Input: part model. Units: mm. Frame: model coordinates. A direction names the side the tool comes from. Give positions to 0.01 mm unless a question says otherwise; leave off trailing zeros. Loops run counter-clockwise (first coordinate to the right, second up) from the corner with the lowest first, then second, coordinate; pieces in that order, holes last. Notation, with made-up numbers: M -38,19.25 L 12,19.25 A35 cw 12,57.25 Z; hole C -34,60 d1. An arc over 180 degrees is marked long. Answer as a JSON object with one key per item and string values. Group by question number.
1) Section query A-A on y = -1.3. Count the separate pieces of the cut face and the enclosed holes in it, plus the area to 3 significant figures.
2) Ray query, L1, parallel to X at y = 0.15, z = 5; L2, parallel to Z at x = 5.1, y = 1.15; L3, parallel to X at y = 0.45, z = 0.75. Return the intervals inside material, ascending.
3) First-contact query: P1, Ø1, axis at y = 1, z = 4, coming from the -X side; P2, Ø2, axis at y = -1, z = 5, coming from the +X side; P3, Ø3, axis at x = 5.1, z = 3.5, coming from the -Y side. Flat tips, straight axial feed; report the tip coordinate or a pass-through.
4) Access query for faces 5 (the flat face through (-2.35, -1, 3)), 6 (the flat face through (3, -2.5, 3)). Directions: +Z, -Z, +X, -X, +Y, -Y. A direction counts if a zero-diameter tool reaches every point of the face in a straight line with its end or side. Return the directions, or none.
5) Draft query along X for faces 1 (the flat face through (2.35, -1, 3)), 2 (the flat face through (-4.35, -1, 3)), 3 (the flat face through (0.9, 2.4, 7)), 4 (the cylindrical face through (6.8, 0.5, 1)). Return one class per face: +X half, -X half, draft (parallel to the pull), parting line (faces both ways), or undercut.
6) Section query B-B on z = 2. Return loops of the section in (x, y), plus the area to 3 significant figures.
7) Section query C-C on x = 5.1. Return loops of the section in (y, z), plus the area to 3 significant figures.
from build123d import *

# Parameters (mm, degrees)
F1_DEPTH = 7
F2_R     = 1.75
F3_DEPTH = 5.85
F4_R     = 3.49999
F5_R     = 3


# Not quite as in the source:
# - a fillet or chamfer is up to 0.001 mm smaller than in the source, because OpenCascade refuses the exact size


with BuildPart() as f1:
    # F0 (on Top) → F1 (new body)
    with BuildSketch(Plane.XY):
        with BuildLine():
            ThreePointArc((-2.35, 0), (0, 2.35), (2.35, 0))
            Line((2.35, 0), (2.35, -2.5))
            Line((2.35, -2.5), (7.85, -2.5))
            Line((7.85, -2.5), (7.85, 3.35))
            Line((7.85, 3.35), (-4.35, 3.35))
            Line((-4.35, 3.35), (-4.35, -2.5))
            Line((-4.35, -2.5), (-2.35, -2.5))
            Line((-2.35, -2.5), (-2.35, 0))
        make_face()
    extrude(amount=F1_DEPTH)

    # F2 (on face) → F3 (cut, through all)
    with BuildSketch(Plane(origin=(0, 3.35, 0), x_dir=(-1, 0, 0), z_dir=(0, 1, 0))):
        with Locations((-5.1, 3.5)):
            Circle(F2_R)
    extrude(amount=-F3_DEPTH, mode=Mode.SUBTRACT)

    # F4 (radius 3.5 in the source; OpenCascade refuses exactly that, so slightly less here)
    f4_edges = [f1.edges().sort_by_distance(p)[0] for p in [
        (7.85, 0.425, 7),
        (7.85, 0.425, 0),
    ]]
    fillet(f4_edges, radius=F4_R)

    # F5
    f5_edges = [f1.edges().sort_by_distance(p)[0] for p in [
        (-4.35, 3.35, 3.5),
    ]]
    fillet(f5_edges, radius=F5_R)


solid = f1.part
Output:
{
 "1": {"separate pieces": "2", "enclosed holes": "1", "area": "37.6 mm^2"},
 "2": {"L1": "x = -4.35 to -2.35, 2.35 to 4.2, 6 to 7.51", "L2": "z = 0.08 to 1.75, 5.25 to 6.92", "L3": "x = -4.35 to -2.31, 2.31 to 6.52"},
 "3": {"P1": "stops at x = -4.35", "P2": "stops at x = 7.81", "P3": "passes through"},
 "4": {"face 5": "+Z, -Z, -Y", "face 6": "+Z, -Z, +X, -X, -Y"},
 "5": {"face 1": "undercut", "face 2": "-X half", "face 3": "draft", "face 4": "+X half"},
 "6": {"outline": "M -4.35,-2.5 L -2.35,-2.5 L -2.35,0 A2.35 cw 2.35,0 L 2.35,-2.5 L 4.2,-2.5 L 4.2,3.35 L -1.35,3.35 A3 ccw -4.35,0.35 Z; M 6,-2.5 L 7.51,-2.5 L 7.51,3.35 L 6,3.35 Z", "area": "36.5 mm^2"},
 "7": {"outline": "M -2.5,0.08 L 3.35,0.08 L 3.35,1.75 L -2.5,1.75 Z; M -2.5,5.25 L 3.35,5.25 L 3.35,6.92 L -2.5,6.92 Z", "area": "19.5 mm^2"}
}
